Geometry check sheet. Reference: drawing and pictorial views, mm from the part's lowest x, y, z. A direction names the side the tool comes from. Give positions to 0.01 mm unless a question says otherwise; leave off trailing zeros. Write each loop counter-clockwise with the first axis right and the second up, starting at its lowest first coordinate (ties: lowest second). Pieces come first, ordered by that corner, then holes.
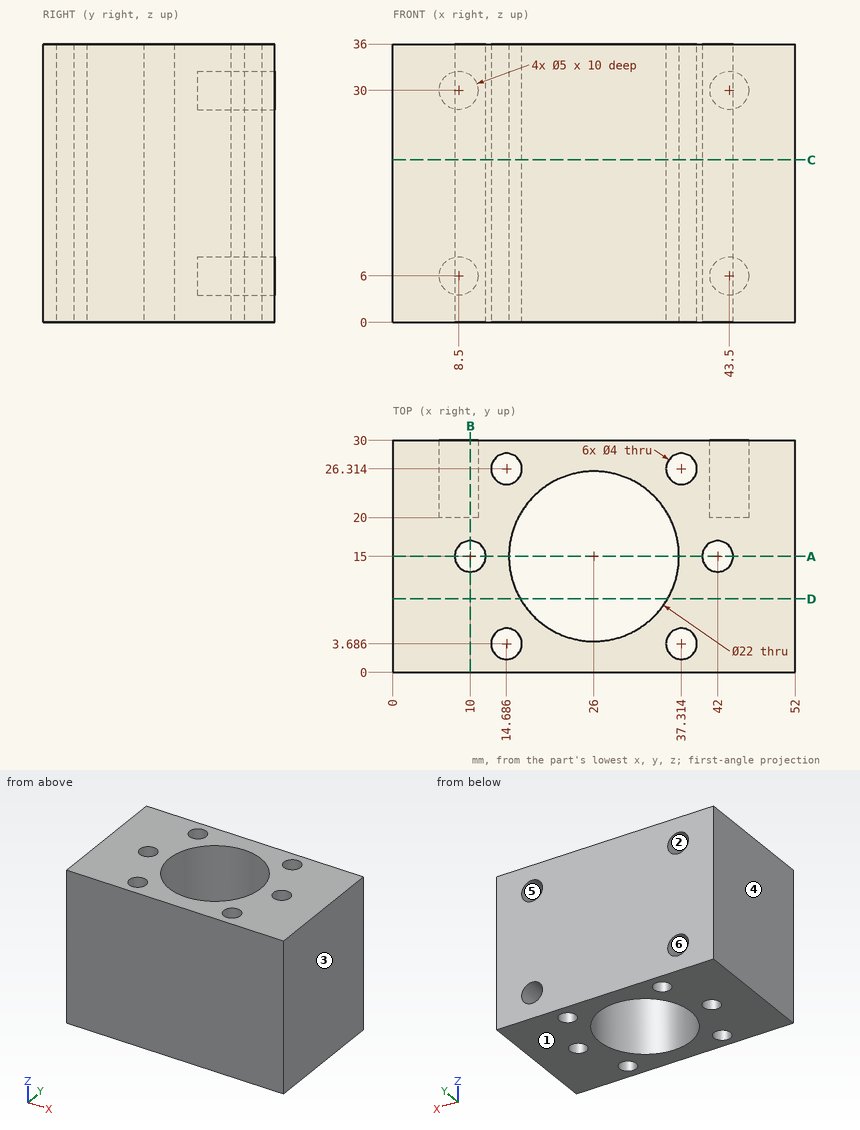
Item 1: Depth check by flat-ended pin: pin 1 (3 mm diameter, centred on x = 8.5, z = 30, fed in from +Y); pin 2 (2.5 mm diameter, centred on x = 37.31, y = 3.69, fed in from -Z). Enter the tip coordinate at first touch or a pass-through.
Answer key:
pin 1: stops at y = 20
pin 2: passes through
Item 2: Sectioned sample at A-A on y = 15. Record the cut outline in (x, z), then the cut area to 3 significant figures.
Answer key:
outline: (0, 0) - (8, 0) - (8, 36) - (0, 36) - close; (12, 0) - (15, 0) - (15, 36) - (12, 36) - close; (37, 0) - (40, 0) - (40, 36) - (37, 36) - close; (44, 0) - (52, 0) - (52, 36) - (44, 36) - close
area: 792 mm2
Item 3: Release check for a two-part mould opening along X. For the marked faces 3, 4, 5 and 6 record: released by +X, released by -X, zero draft, split by the parting line, or undercut.
Answer key:
face 3: released by +X
face 4: released by -X
face 5: undercut
face 6: undercut
Item 4: Sectioned sample at C-C on z = 21. Record the cut outline in (x, y), then the cut area to 3 significant figures.
Answer key:
outline: (0, 0) - (52, 0) - (52, 30) - (0, 30) - close; hole circle Ø4 at (10, 15); hole circle Ø4 at (14.69, 3.69); hole circle Ø4 at (14.69, 26.31); hole circle Ø22 at (26, 15); hole circle Ø4 at (37.31, 3.69); hole circle Ø4 at (37.31, 26.31); hole circle Ø4 at (42, 15)
area: 1,100 mm2
Item 5: Scan lines: line 1 along X through (y, z) = (26.5, 10) (1 decimal); line 2 along Z through (x, y) = (43.5, 26); line 3 along X through (y, z) = (16.75, 22). Record each from-to range of solid material in increasing order.
Answer key:
line 1: x = 0 to 12.7, 16.7 to 35.3, 39.3 to 52
line 2: z = 0 to 3.5, 8.5 to 27.5, 32.5 to 36
line 3: x = 0 to 9.03, 10.97 to 15.14, 36.86 to 41.03, 42.97 to 52
Item 6: Sectioned sample at B-B on x = 10. Record the cut outline in (y, z), then the cut area to 3 significant figures.
Answer key:
outline: (0, 0) - (13, 0) - (13, 36) - (0, 36) - close; (17, 0) - (30, 0) - (30, 4) - (20, 4) - (20, 8) - (30, 8) - (30, 28) - (20, 28) - (20, 32) - (30, 32) - (30, 36) - (17, 36) - close
area: 856 mm2
Item 7: Set-up check for the marked faces 1 and 2: record each of +Z, -Z, +X, -X, +Y, -Y from which the full face is reachable in a straight line by a thin tool's end or side.
Answer key:
face 1: -Z, +X, -X, +Y, -Y
face 2: +Y
Item 8: Sectioned sample at D-D on y = 9.5. Record the cut outline in (x, z).
Answer key:
outline: (0, 0) - (16.47, 0) - (16.47, 36) - (0, 36) - close; (35.53, 0) - (52, 0) - (52, 36) - (35.53, 36) - close
